from build123d import *

# Parameters (mm, degrees)
BOSS_EXTRUDE1_DEPTH           = 50.8
FILLET1_R                     = 50.8
SHELL1_T                      = -2.54
SKETCH2_W                     = 45.72
SKETCH2_H                     = 45.72
CUT_EXTRUDE1_DEPTH            = 50.8
F_97_0_5_DIAMETER_HOLE1_D     = 12.7
F_97_0_5_DIAMETER_HOLE2_D     = 12.7
F_97_0_5_DIAMETER_HOLE2_DEPTH = 12.7
F_97_0_5_DIAMETER_HOLE2_TIP   = 3.815464931


with BuildPart() as part:
    # Sketch1 → Boss-Extrude1 (new body)
    with BuildSketch(Plane.XY):
        Polygon((0, 0), (0, 330.2), (-647.7, 871.912727273), (-647.7, 1244.6), (-698.5, 1244.6), (-698.5, 848.174564223), (-50.8, 306.461836951), (-50.8, 0), align=None)
    extrude(amount=BOSS_EXTRUDE1_DEPTH)

    # Fillet1
    fillet1_edges = [part.edges().sort_by_distance(p)[0] for p in [
        (-50.8, 306.461836951, 25.4),
        (-698.5, 848.174564223, 25.4),
        (-647.7, 871.912727273, 25.4),
        (0, 330.2, 25.4),
    ]]
    fillet(fillet1_edges, radius=FILLET1_R)

    # Shell1
    shell1_openings = [part.faces().sort_by_distance(p)[0] for p in [
        (-673.1, 1244.6, 25.4),
    ]]
    offset(amount=SHELL1_T, openings=shell1_openings, kind=Kind.INTERSECTION)

    # Sketch2 → Cut-Extrude1 (cut)
    with BuildSketch(Plane.XZ):
        with Locations((-25.4, 25.4)):
            Rectangle(SKETCH2_W, SKETCH2_H)
    extrude(amount=-CUT_EXTRUDE1_DEPTH, mode=Mode.SUBTRACT)

    # #97 (0.5) Diameter Hole1 (through all)
    with Locations(Plane(origin=(0, 19.05, 25.4), x_dir=(0, 0, 1), z_dir=(1, 0, 0))):
        with Locations((0, 0), (0, -146.05)):
            Hole(F_97_0_5_DIAMETER_HOLE1_D / 2)

    # #97 (0.5) Diameter Hole2
    with Locations(Plane(origin=(-582.872241676, 751.467711807, 25.4), x_dir=(-0.767076870152, 0.641555200491, 0), z_dir=(-0.641555200491, -0.767076870152, 0))):
        with Locations((-1e-09, 0)):
            Hole(F_97_0_5_DIAMETER_HOLE2_D / 2, depth=F_97_0_5_DIAMETER_HOLE2_DEPTH)
            with Locations((0, 0, -(F_97_0_5_DIAMETER_HOLE2_DEPTH + F_97_0_5_DIAMETER_HOLE2_TIP / 2))):  # 118° drill point
                Cone(0, F_97_0_5_DIAMETER_HOLE2_D / 2, F_97_0_5_DIAMETER_HOLE2_TIP, mode=Mode.SUBTRACT)


solid = part.part
Work out the finished part from the listing and answer in its coordinate system (mm). A direction names the side the tool comes from. Give positions to 0.01 mm unless a question says otherwise; leave off trailing zeros. Loops run counter-clockwise (first coordinate to the right, second up) from the corner with the lowest first, then second, coordinate; pieces in that order, holes last. Notation, with made-up numbers: (82.5, 6.5) - (103.5, 6.5) arc R15 ccw to (103.5, 29.5) - close; hole circle Ø1 at (22.5, -29.5). An arc over 180 degrees is marked (long way). Answer in a Markdown table with one row per item. Add a question column.
Q1. A tool of negligible diameter and unlimited length cuts with its end or side. For faces 1 (the flat face through (-650.24, 1068, 25)), 2 (the flat face through (-647.7, 1068, 25)), 3 (the flat face through (-321.2, 595.53, 25.08)), from which of +Z, -Z, +X, -X, +Y, -Y can it reach the whole face along a straight path? Write none if from no direction.
Q2. The part is cut by section A-A (y = 934.5). Determine the outline of the cut face in (x, z), and give its area (3 significant figures).
Q3. Consider line 1 along X through (y, z) = (1172.5, 37); line 2 along Y through (x, z) = (-471, 21.5); line 3 along X through (y, z) = (628.5, 47). Determine where each line is inside the solid, lowest interval first.
Q4. Each of these flat-tipped pins is pushed along its axis until it touches: P1, Ø14.5, axis at y = 165.1, z = 25.4, coming from the -X side; P2, Ø1, axis at y = 450.5, z = 34.5, coming from the +X side; P3, Ø5, axis at x = -199, z = 45, coming from the +Y side; P4, Ø10, axis at y = 19.05, z = 25.4, coming from the +X side. Where does it stop, or does it pass through?
Q5. The part is cut by section B-B (x = -236). Determine the outline of the cut face in (y, z).
Q6. Determine the mould class of faces 4 (the cylindrical face through (-53.415, 305.6, 25.72)), 5 (the flat face through (-671, 1244.6, 50)), 6 (the flat face through (-377, 625, 50.8)) for opening direction Z: released by +Z, released by -Z, zero draft, split by the parting line, or undercut.
Solution:
| question | item | result |
|---|---|---|
| 1 | face 1 | +Y |
| 1 | face 2 | +Z, -Z, +X, +Y |
| 1 | face 3 | none |
| 2 | outline | (-698.5, 0) - (-647.7, 0) - (-647.7, 50.8) - (-698.5, 50.8) - close; hole (-695.96, 2.54) - (-650.24, 2.54) - (-650.24, 48.26) - (-695.96, 48.26) - close |
| 2 | area | 490 mm² |
| 3 | line 1 | x = -698.5 to -695.96, -650.24 to -647.7 |
| 3 | line 2 | y = 657.9 to 661.21, 720.82 to 724.13 |
| 3 | line 3 | x = -435.85 to -431.89, -360.62 to -356.66 |
| 4 | P1 | stops at x = -50.8 |
| 4 | P2 | stops at x = -143.24 |
| 4 | P3 | stops at y = 498.73 |
| 4 | P4 | passes through |
| 5 | outline | (461.36, 0) - (527.58, 0) - (527.58, 50.8) - (461.36, 50.8) - close; hole (464.67, 2.54) - (524.27, 2.54) - (524.27, 48.26) - (464.67, 48.26) - close |
| 6 | face 4 | undercut |
| 6 | face 5 | zero draft |
| 6 | face 6 | released by +Z |
